```python
from build123d import *

# Parameters (mm, degrees)
EXTRUDE_2_DEPTH     = 4
SKETCH_4_R          = 6.1
SKETCH_4_R_2        = 1.75
CUT_EXTRUDE_1_DEPTH = 39.794329483
SKETCH_5_W          = 5
SKETCH_5_H          = 40
CUT_EXTRUDE_2_DEPTH = 4
FILLET_1_R          = 1.5


with BuildPart() as part:
    # Эскиз1 → Бобышка-Вытянуть2 (new body)
    with BuildSketch(Plane.XY):
        with BuildLine():
            Line((31.5, -20), (-31.5, -20))
            ThreePointArc((-31.5, -20), (-32.560660172, -19.560660172), (-33, -18.5))
            Line((-33, -18.5), (-33, 18.5))
            ThreePointArc((-33, 18.5), (-32.560660172, 19.560660172), (-31.5, 20))
            Line((-31.5, 20), (31.5, 20))
            ThreePointArc((31.5, 20), (32.560660172, 19.560660172), (33, 18.5))
            Line((33, 18.5), (33, -18.5))
            ThreePointArc((33, -18.5), (32.560660172, -19.560660172), (31.5, -20))
        make_face()
    extrude(amount=EXTRUDE_2_DEPTH)

    # Эскиз4 → Вырез-Вытянуть1 (cut, through all)
    with BuildSketch(Plane(origin=(0, 0, 0), x_dir=(-1, 0, 0), z_dir=(0, 0, -1))):
        with Locations((21.7, 0)):
            Circle(SKETCH_4_R)
        with Locations((21.7, -14)):
            Circle(SKETCH_4_R_2)
        with Locations((5.7, -8)):
            Circle(SKETCH_4_R_2)
        with Locations((-9.3, -8)):
            Circle(SKETCH_4_R_2)
        with Locations((-23, -14)):
            Circle(SKETCH_4_R_2)
        with Locations(Location((21.7, 14, 0), (0, 0, 180))):
            Circle(SKETCH_4_R_2)
        with Locations(Location((5.7, 8, 0), (0, 0, 180))):
            Circle(SKETCH_4_R_2)
        with Locations(Location((-9.3, 8, 0), (0, 0, 180))):
            Circle(SKETCH_4_R_2)
        with Locations(Location((-23, 14, 0), (0, 0, 180))):
            Circle(SKETCH_4_R_2)
    extrude(amount=-CUT_EXTRUDE_1_DEPTH, mode=Mode.SUBTRACT)

    # Эскиз5 → Вырез-Вытянуть2 (cut)
    with BuildSketch(Plane(origin=(0, 0, 0), x_dir=(-1, 0, 0), z_dir=(0, 0, -1))):
        Polygon((27.8, 20), (33, 20), (33, -20), (27.8, -20), (27.8, -6.1), (21.7, -6.1), (21.7, 6.1), (27.8, 6.1), align=None)
        with Locations((-30.5, 0)):
            Rectangle(SKETCH_5_W, SKETCH_5_H)
    extrude(amount=-CUT_EXTRUDE_2_DEPTH, mode=Mode.SUBTRACT)

    # Скругление1
    fillet_1_edges = [part.edges().sort_by_distance(p)[0] for p in [
        (28, 20, 2),
        (28, -20, 2),
        (-27.8, 20, 2),
        (-27.8, -20, 2),
    ]]
    fillet(fillet_1_edges, radius=FILLET_1_R)


solid = part.part
```
Part model, mm, in its own coordinate system. A direction names the side the tool comes from. Round coordinates to 2 decimals unless told otherwise and drop trailing zeros. Write each loop counter-clockwise with the first axis right and the second up, starting at its lowest first coordinate (ties: lowest second). Pieces come first, ordered by that corner, then holes. Notation, with made-up numbers: (-7, 59) -> (39, 59) arc R31 cw to (39, 89) -> close; hole circle Ø5 at (9, -5.75). An arc over 180 degrees is marked (long way). Return JSON: item names as keys, results as strings. Group by question number.
Q1. Which spindle directions (+Z, -Z, +X, -X, +Y, -Y) get a long thin tool onto all of the face, cutting with end or side? Do faces 1 (the cylindrical face through (-27.35, 19.57, 2.03)), 2 (the flat face through (-25, 6.1, 2)). Say none if no direction does.
Q2. Mould opens along Y. For faces 3 (the cylindrical face through (21.71, 12.82, 1.97)), 4 (the flat face through (-27.8, -12, 2)), 5 (the cylindrical face through (-27.35, -19.57, 2.03)) say: pulls with the +Y half, pulls with the -Y half, needs draft (parallel to the pull), parting line crosses it, or undercut.
Q3. Saw through at A-A on y = 8. Write the cut outline in (x, z).
Q4. Saw through at C-C on z = 3.4. State how many separate pieces and enclosed holes the cut face has, plus the area to 3 significant figures.
Q5. Saw through at D-D on y = 0. Write the cut outline in (x, z).
Q6. Saw through at B-B on x = -5.7. Write the cut outline in (y, z), plus the area to 3 significant figures.
Q7. Probe L1, parallel to X at y = 8, z = 3.05; L2, parallel to Y at x = 9.3, z = 1.05; L3, parallel to Y at x = -21.7, z = 2.9. List the from-to ranges inside material, lowest first. Write a range as [from, to].
Answer:
{
 "1": {"face 1": "+Z, -Z, -X, +Y", "face 2": "+Z, -Z, -X"},
 "2": {"face 3": "undercut", "face 4": "needs draft", "face 5": "pulls with the -Y half"},
 "3": {"outline": "(-27.8, 0) -> (-7.45, 0) -> (-7.45, 4) -> (-27.8, 4) -> close; (-3.95, 0) -> (7.55, 0) -> (7.55, 4) -> (-3.95, 4) -> close; (11.05, 0) -> (28, 0) -> (28, 4) -> (11.05, 4) -> close"},
 "4": {"separate pieces": "1", "enclosed holes": "8", "area": "2,020 mm2"},
 "5": {"outline": "(-15.6, 0) -> (28, 0) -> (28, 4) -> (-15.6, 4) -> close"},
 "6": {"outline": "(-20, 0) -> (-9.75, 0) -> (-9.75, 4) -> (-20, 4) -> close; (-6.25, 0) -> (6.25, 0) -> (6.25, 4) -> (-6.25, 4) -> close; (9.75, 0) -> (20, 0) -> (20, 4) -> (9.75, 4) -> close", "area": "132 mm2"},
 "7": {"L1": "[-27.8, -7.45], [-3.95, 7.55], [11.05, 28]", "L2": "[-20, -9.75], [-6.25, 6.25], [9.75, 20]", "L3": "[-20, -15.75], [-12.25, -6.1], [6.1, 12.25], [15.75, 20]"}
}
